from build123d import *

# Parameters (mm, degrees)
SKETCH1_W           = 13
SKETCH1_H           = 2
SKETCH1_W_2         = 10.5
SKETCH1_H_2         = 1
BOSS_EXTRUDE1_DEPTH = 1
CUT_EXTRUDE2_DEPTH  = 1


with BuildPart() as part:
    # Sketch1 → Boss-Extrude1 (new body)
    with BuildSketch(Plane(origin=(0, 0, 0), x_dir=(1, 0, 0), z_dir=(0, 1, 0))):
        Rectangle(SKETCH1_W, SKETCH1_H)
        with Locations((-0.25, 0)):
            Rectangle(SKETCH1_W_2, SKETCH1_H_2, mode=Mode.SUBTRACT)
    extrude(amount=BOSS_EXTRUDE1_DEPTH)

    # Sketch2 → Cut-Extrude2 (cut)
    with BuildSketch(Plane.ZY.offset(6.5)):
        with BuildLine():
            Line((0.15, 0.5), (0.15, 0.8))
            Line((0.15, 0.8), (0.275, 0.8))
            Line((0.275, 0.8), (0.275, 1))
            Line((0.275, 1), (0.15, 1))
            Line((0.15, 1), (-0.15, 1))
            Line((-0.15, 1), (-0.275, 1))
            Line((-0.275, 1), (-0.275, 0.8))
            Line((-0.275, 0.8), (-0.15, 0.8))
            Line((-0.15, 0.8), (-0.15, 0.5))
            ThreePointArc((-0.15, 0.5), (0, 0.35), (0.15, 0.5))
        make_face()
    extrude(amount=-CUT_EXTRUDE2_DEPTH, mode=Mode.SUBTRACT)


solid = part.part
Read the model definition and answer for the solid it produces. Units are mm, in the model's axes. A direction names the side the tool comes from. Round coordinates to 2 decimals unless told otherwise and drop trailing zeros. Loops run counter-clockwise (first coordinate to the right, second up) from the corner with the lowest first, then second, coordinate; pieces in that order, holes last.
Q1. Section B-B on y = 0.2 is taken. Write down the section's boundary in (x, z).
Q2. Section C-C on z = 0 is taken. Write down the section's boundary in (x, y).
Q3. Consider probe 1 along Z at (x, y) = (1.75, 0.3); probe 2 along X at (y, z) = (0.75, 0.2); probe 3 along X at (y, z) = (0.8, 0). Determine where each line is inside the solid, lowest interval first.
Q4. Which of the six approach directions +Z, -Z, +X, -X, +Y, -Y give full straight-line access (tool end or side, diameter ignored) to faces 1 (the face through (-0.1, 0, -0.7)), 2 (the face through (5, 0.5, 0))?
Q5. Determine the mould class of faces 3 (the face through (-0.3, 0.5, 0.5)), 4 (the face through (-0.3, 0.5, -0.5)), 5 (the face through (-0.1, 0.5, 1)), 6 (the face through (-0.1, 0.5, -1)) for opening direction Z: released by +Z, released by -Z, zero draft, split by the parting line, or undercut.
Q6. Section A-A on x = 0 is taken. Write down the section's boundary in (y, z).
Output:
1. outline: (-6.5, -1) - (6.5, -1) - (6.5, 1) - (-6.5, 1) - close; hole (-5.5, -0.5) - (5, -0.5) - (5, 0.5) - (-5.5, 0.5) - close
2. outline: (-6.5, 0) - (-5.5, 0) - (-5.5, 0.35) - (-6.5, 0.35) - close; (5, 0) - (6.5, 0) - (6.5, 1) - (5, 1) - close
3. probe 1: z = -1 to -0.5, 0.5 to 1
3. probe 2: x = -6.5 to -5.5, 5 to 6.5
3. probe 3: x = 5 to 6.5
4. face 1: +Z, -Z, +X, -X, -Y
4. face 2: +Y, -Y
5. face 3: undercut
5. face 4: undercut
5. face 5: released by +Z
5. face 6: released by -Z
6. outline: (0, -1) - (1, -1) - (1, -0.5) - (0, -0.5) - close; (0, 0.5) - (1, 0.5) - (1, 1) - (0, 1) - close
